Autodesk Inventor part; units mm, degrees
ref_plane "作業平面1" through (0, 0, 0) normal (0, 0, 1) x (1, 0, 0)
ref_plane "YZ Plane" through (0, 0, 0) normal (1, 0, 0) x (0, 1, 0)
ref_plane "XZ Plane" through (0, 0, 0) normal (0, 1, 0) x (-1, 0, 0)
ref_plane "作業平面1" through (0, 0, 0) normal (0, 0, 1) x (1, 0, 0)
sketch "スケッチ2" plane through (0, 0, 0) normal (0, 0, 1) x (1, 0, 0)
  line L0 (0, 0) -> (7.35, 0) construction
  line L1 (7.35, 0) -> (7.35, 50) construction
  line L2 (0, 50) -> (7.35, 50) construction
  line L3 (0, 0) -> (0, 50) construction
  line L4 (-0.5, 0) -> (-0.5, 50) construction
  line L5 (19.5, 0) -> (19.5, 50) construction
  line L6 (139.5, 0) -> (139.5, -3) construction
  line L7 (139.5, 0) -> (4.5, 0) construction
  line L8 (4.5, -3) -> (4.5, 0) construction
  line L9 (139.5, -3) -> (4.5, -3) construction
  line L10 (139.5, 53) -> (139.5, 50) construction
  line L11 (4.5, 53) -> (139.5, 53) construction
  line L12 (4.5, 50) -> (4.5, 53) construction
  line L13 (4.5, 50) -> (139.5, 50) construction
  line L14 (-0.632, 5) -> (-130.632, 5) construction
  line L15 (-0.632, 45) -> (-130.632, 45) construction
  line L16 (-20.5, 10) -> (-20.5, 40)
  line L17 (-20.5, 40) -> (-0.5, 40)
  line L18 (-0.5, 40) -> (-0.5, 5)
  circle A0 centre (14.5, 15) radius 3.3
  circle A1 centre (14.5, 35) radius 3.3
  circle A2 centre (-10.5, 25) radius 3.3
  circle A3 centre (-10.5, 25) radius 3.3
  line L19 (-20.5, 10) -> (-0.5, 10)
  line L20 (-0.5, 0) -> (29.5, 0)
  line L21 (29.5, 0) -> (29.5, 50)
  line L22 (29.5, 50) -> (-0.5, 50)
  line L23 (-0.5, 50) -> (-0.5, 0)
  point P0 (9.5, 35)
  point P1 (-0.5, 40)
  point P2 (-0.5, 5)
  dimension "d1" = 20
  dimension "d2" = 30
  dimension "d4" = 50
  dimension "d5" = 15
  dimension "d13" = 6.6
  dimension "d17" = 6.6
  dimension "d19" = 10
  dimension "d20" = 6.6
  dimension "d22" = 10
  dimension "d23" = 6.6
  dimension "d25" = 15
  dimension "d27" = 10
  dimension "d29" = 15
  dimension "d30" = 15
  dimension "d31" = 30
  dimension "d32" = 50
  dimension "d33" = 15
  dimension "d34" = 15
extrude "押し出し1" add sketch "スケッチ2" along normal blind 3
fillet "フィレット1" radius 5 6 edges at (-20.5, 10, 1.5) (-20.5, 40, 1.5) (-0.5, 0, 1.5) (29.5, 0, 1.5) (-0.5, 50, 1.5) (29.5, 50, 1.5)
equation "\"d22\" = d19"
equation "\"d23\" = d13"
equation "\"d27\" = -0.5 * d2 + 0.5 * d28"
equation "\"d29\" = 0.5 * d2"
equation "\"d30\" = d29"
equation "\"d33\" = 0.5 * d31"
equation "\"d34\" = d33"
properties part number "bogie_mount" material "アルミニウム 6061"
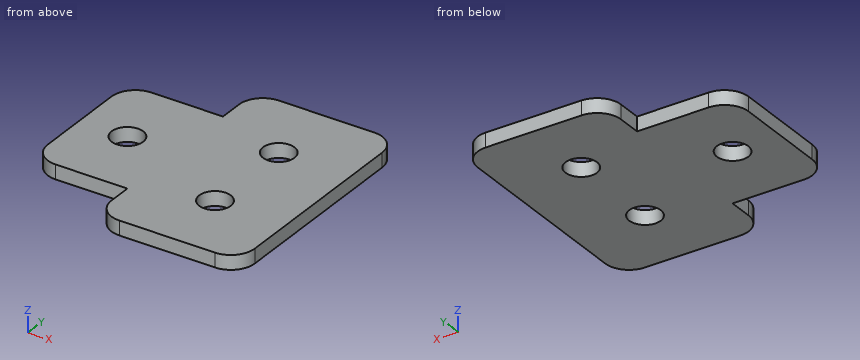
The model under review builds one solid part; all positions refer to its coordinate system, in mm. Coordinates: 2 decimals unless noted, no trailing zeros. Write each loop counter-clockwise with the first axis right and the second up, starting at its lowest first coordinate (ties: lowest second). Pieces come first, ordered by that corner, then holes. Notation, with made-up numbers: (14.5, 28.25) - (18.5, 28.25) arc R16 cw to (18.5, 55.25) - close; hole circle Ø7 at (38.5, 53). An arc over 180 degrees is marked (long way). Answer as CSV lines item,"result".
(1) We need section A-A (x = -10.5). Give the boundary of the cut face in (y, z).
Data:
outline,"(10, 0) - (21.7, 0) - (21.7, 3) - (10, 3) - close; (28.3, 0) - (40, 0) - (40, 3) - (28.3, 3) - close"
(2) For line 1 along Y through (x, z) = (14.5, 0.6); line 2 along Y through (x, z) = (-10.5, 2.15); line 3 along Y through (x, z) = (13.5, 0.35), list the stretches that pass through material, from the lowest coordinate up. Write a range as [from, to].
Data:
line 1,"y = [0, 11.7], [18.3, 31.7], [38.3, 50]"
line 2,"y = [10, 21.7], [28.3, 40]"
line 3,"y = [0, 11.86], [18.14, 31.86], [38.14, 50]"
(3) We need section D-D (z = 1.2). Give the boundary of the cut face in (x, y), plus the area to 3 significant figures.
Data:
outline,"(-20.5, 15) arc R5 ccw to (-15.5, 10) - (-0.5, 10) - (-0.5, 5) arc R5 ccw to (4.5, 0) - (24.5, 0) arc R5 ccw to (29.5, 5) - (29.5, 45) arc R5 ccw to (24.5, 50) - (4.5, 50) arc R5 ccw to (-0.5, 45) - (-0.5, 40) - (-15.5, 40) arc R5 ccw to (-20.5, 35) - close; hole circle Ø6.6 at (-10.5, 25); hole circle Ø6.6 at (14.5, 15); hole circle Ø6.6 at (14.5, 35)"
area,"1,970 mm2"
(4) We need section B-B (y = 25). Give the boundary of the cut face in (x, z), plus the area to 3 significant figures.
Data:
outline,"(-20.5, 0) - (-13.8, 0) - (-13.8, 3) - (-20.5, 3) - close; (-7.2, 0) - (29.5, 0) - (29.5, 3) - (-7.2, 3) - close"
area,"130 mm2"
(5) We need section C-C (x = 14.5). Give the boundary of the cut face in (y, z).
Data:
outline,"(0, 0) - (11.7, 0) - (11.7, 3) - (0, 3) - close; (18.3, 0) - (31.7, 0) - (31.7, 3) - (18.3, 3) - close; (38.3, 0) - (50, 0) - (50, 3) - (38.3, 3) - close"
(6) Clearance check with flat-ended pins moving along their axes: pin 1 Ø1.5 at (x, z) = (-9, 1.5) entering from -Y; pin 2 Ø1.5 at (y, z) = (42.5, 2) entering from -X; pin 3 Ø10.5 at (x, y) = (-10.5, 25) entering from -Z; pin 4 Ø4 at (x, y) = (14.5, 35) entering from -Z. State where each tip first meets the part, or that it passes through.
Data:
pin 1,"stops at y = 10"
pin 2,"stops at x = -0.5"
pin 3,"stops at z = 0"
pin 4,"passes through"
